For this review, take the finished solid that the model builds, in its own axes (mm). Face numbers are marked on the shaded views. A direction names the side the tool comes from. Round coordinates to 2 decimals unless told otherwise and drop trailing zeros. Loops run counter-clockwise (first coordinate to the right, second up) from the corner with the lowest first, then second, coordinate; pieces in that order, holes last. Notation, with made-up numbers: (33, 58.25) -> (41, 58.25) arc R25 cw to (41, 81.25) -> close; hole circle Ø4 at (87.5, 87.25). An arc over 180 degrees is marked (long way). One line per question, with ' | ' between items. Start each with the question number.
1. Wall thickness on line 1 along Y through (x, z) = (0, 2.5); line 2 along Y through (x, z) = (6.5, 4.25); line 3 along X through (y, z) = (2, 3.75): over which ranges is each line inside the solid? List them lowest first.
2. For pin 1 Ø3 at (x, z) = (0.5, 5) entering from +Y; pin 2 Ø2 at (x, z) = (-13, 2.5) entering from +Y; pin 3 Ø2 at (y, z) = (-4.5, 3.5) entering from +X, all flat-tipped, find the tip position at first contact; note any pin that passes through.
3. Consider section C-C (z = 6.5). Write out the cut boundary in (x, y), and give its area (3 significant figures).
4. Consider section D-D (z = 1.5). Write out the cut boundary in (x, y).
5. Consider section A-A (y = 0). Write out the cut boundary in (x, z).
6. Draft analysis for pull direction Y (two halves, no side actions). For the marked faces 1, 2, 3 and 4, state which applies: pulls with the +Y half, pulls with the -Y half, needs draft (parallel to the pull), parting line crosses it, or undercut.
7. For the marked faces 5, 6, 7, 8 and 9, list the 3-axis set-ups (+Z, -Z, +X, -X, +Y, -Y) from which the entire face can be reached by the end or side of a thin tool; tool diameter is ignored.
```python
from build123d import *

# Parameters (mm, degrees)
SKETCH1_R          = 25
SKETCH1_R_2        = 16.25
EXTRUDE1_DEPTH     = 8
CUT_EXTRUDE1_DEPTH = 9
CIRPATTERN1_COUNT  = 4


with BuildPart() as part:
    # Sketch1 → Extrude1 (new body)
    with BuildSketch(Plane.XY):
        Circle(SKETCH1_R)
        Circle(SKETCH1_R_2, mode=Mode.SUBTRACT)
    extrude(amount=EXTRUDE1_DEPTH)

    # Sketch2 → Cut-Extrude1 (cut, through all)
    with BuildSketch(Plane.XY.offset(8)):
        with BuildLine():
            Line((15.02869733, 19.978444798), (12.869343418, 17.819090886))
            Line((12.869343418, 17.819090886), (17.819090886, 12.869343418))
            Line((17.819090886, 12.869343418), (19.978444798, 15.02869733))
            ThreePointArc((19.978444798, 15.02869733), (17.67766953, 17.67766953), (15.02869733, 19.978444798))
        make_face()
    cut_extrude1 = extrude(amount=-CUT_EXTRUDE1_DEPTH, mode=Mode.SUBTRACT)

    # CirPattern1: Cut-Extrude1 ×4 about axis
    cirpattern1_axis = Axis((0, 0, 0), (0, 0, 1))
    for i in range(1, CIRPATTERN1_COUNT):
        add(cut_extrude1.rotate(cirpattern1_axis, i * 360 / CIRPATTERN1_COUNT), mode=Mode.SUBTRACT)

    # Sketch3 → Cut-Revolve1 (revolve, cut)
    with BuildSketch(Plane(origin=(0, 0, 0), x_dir=(1, 0, 0), z_dir=(0, 1, 0))):
        Polygon((25, 0), (21.5, 0), (25, -2.272926576), align=None)
    revolve(axis=Axis((0, 0, 0), (0, 0, -1)), mode=Mode.SUBTRACT)


solid = part.part
```
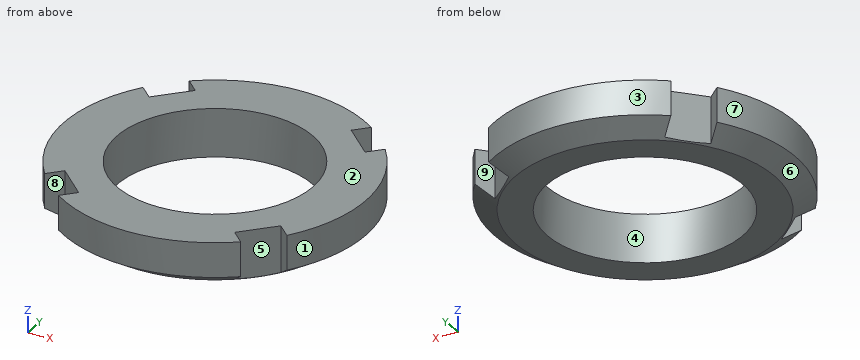
Answer block:
1) line 1: y = -25 to -16.25, 16.25 to 25 | line 2: y = -24.14 to -14.89, 14.89 to 24.14 | line 3: x = -24.92 to -16.13, 16.13 to 24.92
2) pin 1: stops at y = 25 | pin 2: stops at y = 21.93 | pin 3: stops at x = 24.75
3) outline: (-19.98, -15.03) -> (-17.82, -12.87) -> (-12.87, -17.82) -> (-15.03, -19.98) arc R25 ccw to (15.03, -19.98) -> (12.87, -17.82) -> (17.82, -12.87) -> (19.98, -15.03) arc R25 ccw to (19.98, 15.03) -> (17.82, 12.87) -> (12.87, 17.82) -> (15.03, 19.98) arc R25 ccw to (-15.03, 19.98) -> (-12.87, 17.82) -> (-17.82, 12.87) -> (-19.98, 15.03) arc R25 ccw to start; hole circle Ø32.5 at (0, 0) | area: 1,040 mm2
4) outline: (-19.13, -14.18) -> (-17.82, -12.87) -> (-12.87, -17.82) -> (-14.18, -19.13) arc R23.81 ccw to (14.18, -19.13) -> (12.87, -17.82) -> (17.82, -12.87) -> (19.13, -14.18) arc R23.81 ccw to (19.13, 14.18) -> (17.82, 12.87) -> (12.87, 17.82) -> (14.18, 19.13) arc R23.81 ccw to (-14.18, 19.13) -> (-12.87, 17.82) -> (-17.82, 12.87) -> (-19.13, 14.18) arc R23.81 ccw to start; hole circle Ø32.5 at (0, 0)
5) outline: (-25, 2.27) -> (-21.5, 0) -> (-16.25, 0) -> (-16.25, 8) -> (-25, 8) -> close; (16.25, 0) -> (21.5, 0) -> (25, 2.27) -> (25, 8) -> (16.25, 8) -> close
6) face 1: parting line crosses it | face 2: needs draft | face 3: pulls with the +Y half | face 4: undercut
7) face 5: +Z, -Z | face 6: -Z | face 7: +Z, -Z, -X | face 8: +Z, -Z, -Y | face 9: +Z, -Z, +Y
